Source: CAD feature listing. Evaluate the final solid. Frame: model axes, mm. A direction names the side the tool comes from. Round coordinates to 2 decimals unless told otherwise and drop trailing zeros. Loops run counter-clockwise (first coordinate to the right, second up) from the corner with the lowest first, then second, coordinate; pieces in that order, holes last. Notation, with made-up numbers: (88.25, 35.25) - (103.25, 35.25) arc R26 cw to (103.25, 50.25) - close; hole circle Ø1 at (-36, 70.25). An arc over 180 degrees is marked (long way). Write item = value, one per line. Start each with the question number.
from build123d import *

# Parameters (mm, degrees)
CUT_EXTRUDE1_DEPTH = 17
CHAMFER1_SIZE      = 0.288675135
CHAMFER1_SIZE_2    = 0.5
CHAMFER2_SIZE      = 0.5
CHAMFER2_SIZE2     = 0.288675135


with BuildPart() as part:
    # Sketch2 → Revolve1 (revolve)
    with BuildSketch(Plane.XY):
        Polygon((0, 0), (-10, 0), (-10, 4), (0, 4), (0, 6.5), (1.5, 6.5), (1.5, 4), (28, 4), (28, 0), align=None)
    revolve(axis=Axis((28, 0, 0), (-1, 0, 0)))

    # Sketch3 → Cut-Extrude1 (cut)
    with BuildSketch(Plane(origin=(28, 0, 0), x_dir=(0, 0, -1), z_dir=(1, 0, 0))):
        with BuildLine():
            Line((-2, 3.464101615), (2, 3.464101615))
            ThreePointArc((2, 3.464101615), (0, 4), (-2, 3.464101615))
        make_face()
        with BuildLine():
            Line((2, 3.464101615), (4, 0))
            ThreePointArc((4, 0), (3.464101615, 2), (2, 3.464101615))
        make_face()
        with BuildLine():
            Line((-4, 0), (-2, 3.464101615))
            ThreePointArc((-2, 3.464101615), (-3.464101615, 2), (-4, 0))
        make_face()
        with BuildLine():
            ThreePointArc((-4, 0), (-3.464101615, -2), (-2, -3.464101615))
            Line((-2, -3.464101615), (-4, 0))
        make_face()
        with BuildLine():
            ThreePointArc((-2, -3.464101615), (0, -4), (2, -3.464101615))
            Line((2, -3.464101615), (-2, -3.464101615))
        make_face()
        with BuildLine():
            ThreePointArc((2, -3.464101615), (3.464101615, -2), (4, 0))
            Line((4, 0), (2, -3.464101615))
        make_face()
    extrude(amount=-CUT_EXTRUDE1_DEPTH, mode=Mode.SUBTRACT)

    # Chamfer1
    # the kernel refuses this chamfer: 0.5, 0.288675135 mm, written as the material it takes off along each edge
    with BuildSketch(Plane(origin=(11, 0, 0), x_dir=(0, -0.8660254037844389, -0.49999999999999956), z_dir=(0, -0.49999999999999956, 0.8660254037844389))) as chamfer1_piece_1_section:
        Polygon((4, -CHAMFER1_SIZE * 0.999999998596), (4 - CHAMFER1_SIZE_2, 0), (4, 0), align=None)
    chamfer1_piece_1 = revolve(axis=Axis((11, 0, 0), (1, 0, 0)), revolution_arc=60, mode=Mode.PRIVATE)
    chamfer1_piece_1 = split(chamfer1_piece_1, bisect_by=Plane(origin=(10.787249311, -3.461547111, -2.001474844), z_dir=(0, -0.4999999999999996, -0.8660254037844389)), keep=Keep.TOP, mode=Mode.PRIVATE)
    add(chamfer1_piece_1, mode=Mode.SUBTRACT)
    with BuildSketch(Plane(origin=(11, 0, 0), x_dir=(0, 0, 1), z_dir=(0, 1, 0))) as chamfer1_piece_2_section:
        Polygon((4, -CHAMFER1_SIZE * 0.999999998596), (4 - CHAMFER1_SIZE_2, 0), (4, 0), align=None)
    chamfer1_piece_2 = revolve(axis=Axis((11, 0, 0), (1, 0, 0)), revolution_arc=60, mode=Mode.PRIVATE)
    chamfer1_piece_2 = split(chamfer1_piece_2, bisect_by=Plane(origin=(10.787249311, -0.002554504, 3.998525156), z_dir=(0, -0.4999999999999999, 0.8660254037844387)), keep=Keep.TOP, mode=Mode.PRIVATE)
    add(chamfer1_piece_2, mode=Mode.SUBTRACT)
    with BuildSketch(Plane(origin=(11, 0, 0), x_dir=(0, 1, 0), z_dir=(0, 0, -1))) as chamfer1_piece_3_section:
        Polygon((4, -CHAMFER1_SIZE * 0.999999998596), (4 - CHAMFER1_SIZE_2, 0), (4, 0), align=None)
    chamfer1_piece_3 = revolve(axis=Axis((11, 0, 0), (1, 0, 0)), revolution_arc=30, mode=Mode.PRIVATE)
    chamfer1_piece_3 = split(chamfer1_piece_3, bisect_by=Plane(origin=(10.898935311, 3.464101615, 0.855614375), z_dir=(0, 1, 0)), keep=Keep.TOP, mode=Mode.PRIVATE)
    add(chamfer1_piece_3, mode=Mode.SUBTRACT)
    with BuildSketch(Plane(origin=(11, 0, 0), x_dir=(0, 0, -1), z_dir=(0, -1, 0))) as chamfer1_piece_4_section:
        Polygon((4, -CHAMFER1_SIZE * 0.999999998596), (4 - CHAMFER1_SIZE_2, 0), (4, 0), align=None)
    chamfer1_piece_4 = revolve(axis=Axis((11, 0, 0), (1, 0, 0)), revolution_arc=60, mode=Mode.PRIVATE)
    chamfer1_piece_4 = split(chamfer1_piece_4, bisect_by=Plane(origin=(10.787249311, 0.002554504, -3.998525156), z_dir=(0, 0.49999999999999983, -0.8660254037844388)), keep=Keep.TOP, mode=Mode.PRIVATE)
    add(chamfer1_piece_4, mode=Mode.SUBTRACT)
    with BuildSketch(Plane(origin=(11, 0, 0), x_dir=(0, 0.8660254037844386, 0.5000000000000003), z_dir=(0, 0.5000000000000003, -0.8660254037844386))) as chamfer1_piece_5_section:
        Polygon((4, -CHAMFER1_SIZE * 0.999999998596), (4 - CHAMFER1_SIZE_2, 0), (4, 0), align=None)
    chamfer1_piece_5 = revolve(axis=Axis((11, 0, 0), (1, 0, 0)), revolution_arc=60, mode=Mode.PRIVATE)
    chamfer1_piece_5 = split(chamfer1_piece_5, bisect_by=Plane(origin=(10.787249311, 3.461547111, 2.001474844), z_dir=(0, 0.5000000000000001, 0.8660254037844386)), keep=Keep.TOP, mode=Mode.PRIVATE)
    add(chamfer1_piece_5, mode=Mode.SUBTRACT)
    with BuildSketch(Plane(origin=(11, 0, 0), x_dir=(0, -0.8660254037844388, 0.4999999999999997), z_dir=(0, 0.4999999999999997, 0.8660254037844388))) as chamfer1_piece_6_section:
        Polygon((4, -CHAMFER1_SIZE * 0.999999998596), (4 - CHAMFER1_SIZE_2, 0), (4, 0), align=None)
    chamfer1_piece_6 = revolve(axis=Axis((11, 0, 0), (1, 0, 0)), revolution_arc=60, mode=Mode.PRIVATE)
    chamfer1_piece_6 = split(chamfer1_piece_6, bisect_by=Plane(origin=(10.787249311, -3.464101615, 1.997050313), z_dir=(0, -1, 0)), keep=Keep.TOP, mode=Mode.PRIVATE)
    add(chamfer1_piece_6, mode=Mode.SUBTRACT)
    with BuildSketch(Plane(origin=(11, 0, 0), x_dir=(0, 0.8660254037844385, -0.5000000000000003), z_dir=(0, -0.5000000000000003, -0.8660254037844385))) as chamfer1_piece_7_section:
        Polygon((4, -CHAMFER1_SIZE * 0.999999998596), (4 - CHAMFER1_SIZE_2, 0), (4, 0), align=None)
    chamfer1_piece_7 = revolve(axis=Axis((11, 0, 0), (1, 0, 0)), revolution_arc=30, mode=Mode.PRIVATE)
    chamfer1_piece_7 = split(chamfer1_piece_7, bisect_by=Plane(origin=(10.787249311, 3.464101615, -1.997050313), z_dir=(0, 1, 0)), keep=Keep.TOP, mode=Mode.PRIVATE)
    add(chamfer1_piece_7, mode=Mode.SUBTRACT)

    # Chamfer2
    chamfer2_edges = [part.edges().sort_by_distance(p)[0] for p in [
        (28, -1.732050808, -3),
        (28, -1.732050808, 3),
        (28, 3.464101615, 0),
        (28, 1.732050808, -3),
        (28, 1.732050808, 3),
        (28, -3.464101615, 0),
    ]]
    chamfer2_side = [part.faces().sort_by_distance(p)[0] for p in [
        (28, 0, 0),
    ]]
    chamfer(chamfer2_edges, length=CHAMFER2_SIZE, length2=CHAMFER2_SIZE2, reference=chamfer2_side[0])


solid = part.part
(1) Pin query (flat end, axial travel): P1, Ø1.5, axis at x = 0, z = -5, coming from the -Y side; P2, Ø3, axis at y = 4, z = 5, coming from the -X side; P3, Ø0.6, axis at y = 1.5, z = -3, coming from the +X side. Return the tip coordinate at first contact, or that it passes through.
(2) Cut plane D-D (x = -3). Output: boundary loops of the cut face in (y, z), and give its area (3 significant figures).
(3) Material intervals for line 1 along X through (y, z) = (-0.75, 3); line 2 along X through (y, z) = (3.5, -5); line 3 along Y through (x, z) = (23, 3.25), sorted ascending. Write a range as from..to.
(4) Cut plane B-B (x = 19.5). Output: boundary loops of the cut face in (y, z), and give its area (3 significant figures).
(5) Access query for faces 1 (the face through (0, -3, -3)), 2 (the face through (1.5, 3, -3)), 3 (the face through (-10, 0, 0)). Directions: +Z, -Z, +X, -X, +Y, -Y. A direction counts if a zero-diameter tool reaches every point of the face in a straight line with its end or side. Return the directions, or none.
(6) Cut plane C-C (y = 5.5). Output: boundary loops of the cut face in (x, z).
Solution:
q1.P1 = -4.92
q1.P2 = 0
q1.P3 = 27.95
q2.outline = circle Ø8 at (0, 0)
q2.area = 50.3 mm^2
q3.line_1 = -10..27.99
q3.line_2 = 0..1.5
q3.line_3 = -1.3..1.3
q4.outline = (-3.46, -2) - (0, -4) - (3.46, -2) - (3.46, 2) - (0, 4) - (-3.46, 2) - close
q4.area = 41.6 mm^2
q5.face_1 = -X
q5.face_2 = +X
q5.face_3 = +Z, -Z, -X, +Y, -Y
q6.outline = (0, -3.46) - (1.5, -3.46) - (1.5, 3.46) - (0, 3.46) - close
